Read the model definition and answer for the solid it produces. Units are mm, in the model's axes. Face numbers are marked on the shaded views. A direction names the side the tool comes from. Round coordinates to 2 decimals unless told otherwise and drop trailing zeros. Order: outer loops, then holes, each group sorted by start corner. A loop starts at its lowest first (then second) coordinate and runs counter-clockwise, first axis right, second up. Notation, with made-up numbers: (-23.75, -2.5) - (8.25, -2.5) arc R25 cw to (8.25, 16.5) - close; hole circle Ø6 at (41, 8). An arc over 180 degrees is marked (long way). Answer as a JSON object with one key per item and string values. Group by question number.
Q1. A cutting plane is placed at B-B on y = 0. Determine the outline of the cut face in (x, z).
Q2. Given pin 1 Ø3 at (x, z) = (0.5, -7) entering from -Y; pin 2 Ø1.5 at (y, z) = (-1.5, -22.5) entering from +X; pin 3 Ø1.5 at (y, z) = (1.5, -12) entering from -X, each flat-ended and moving along its own axis, determine where each tip first touches the part or whether it passes through.
Q3. A tool of negligible diameter and unlimited length cuts with its end or side. For the marked faces 1 and 2, from which of +Z, -Z, +X, -X, +Y, -Y can it reach the whole face along a straight path? Write none if from no direction.
Q4. The mould has two halves that part along Y. Classify the marked faces 3, 4 and 5: pulls with the +Y half, pulls with the -Y half, needs draft (parallel to the pull), parting line crosses it, or undercut.
Q5. Consider line 1 (Y direction, x = 0, z = -25); line 2 (Z direction, x = -0.25, y = -3); line 3 (Z direction, x = -3.5, y = 1.5). Determine where each line is inside the solid, lowest interval first.
Q6. A cutting plane is placed at D-D on z = -25. Determine the outline of the cut face in (x, y).
Q7. A cutting plane is placed at A-A on x = 0. Determine the outline of the cut face in (y, z).
Q8. A cutting plane is placed at C-C on z = -4. Determine the outline of the cut face in (x, y).
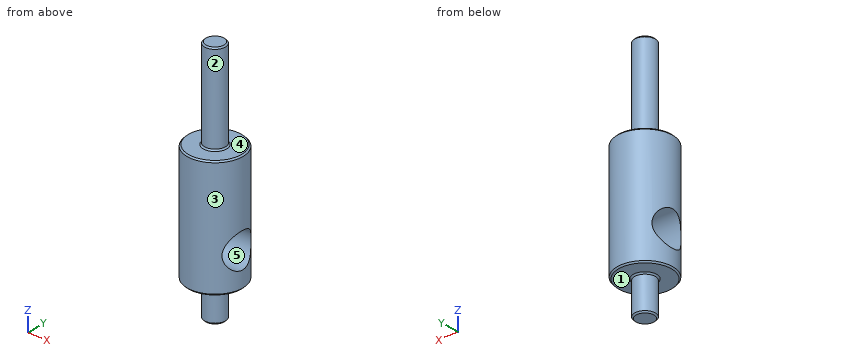
```python
from build123d import *

# Parameters (mm, degrees)
SKETCH1_R               = 1.5
BOSS_EXTRUDE1_DEPTH     = 13
SKETCH2_R               = 4
BOSS_EXTRUDE2_DEPTH     = 17
SKETCH3_R               = 1.5
BOSS_EXTRUDE3_DEPTH     = 5
CUT_EXTRUDE1_DEPTH      = 36.454195802
CUT_EXTRUDE1_DEPTH_BACK = 36.454195802
SKETCH4_R               = 2.5
CHAMFER1_SIZE           = 0.2


with BuildPart() as part:
    # Sketch1 → Boss-Extrude1 (new body)
    with BuildSketch(Plane.XY):
        Circle(SKETCH1_R)
    extrude(amount=-BOSS_EXTRUDE1_DEPTH)

    # Sketch2 → Boss-Extrude2 (add)
    with BuildSketch(Plane(origin=(0, 0, -13), x_dir=(-1, 0, 0), z_dir=(0, 0, -1))):
        Circle(SKETCH2_R)
    extrude(amount=BOSS_EXTRUDE2_DEPTH)

    # Sketch3 → Boss-Extrude3 (add)
    with BuildSketch(Plane(origin=(0, 0, -30), x_dir=(-1, 0, 0), z_dir=(0, 0, -1))):
        with Locations(Location((0, 0, 0), (0, 0, 180))):
            Circle(SKETCH3_R)
    extrude(amount=BOSS_EXTRUDE3_DEPTH)

    # Sketch4 → Cut-Extrude1 (cut, two sides: drawn at the far end of the back side and taken through both)
    with BuildSketch(Plane(origin=(0, 0, 0), x_dir=(0, 0, -1), z_dir=(1, 0, 0)).offset(-CUT_EXTRUDE1_DEPTH_BACK)):
        with Locations((25, 0)):
            Circle(SKETCH4_R)
    extrude(amount=CUT_EXTRUDE1_DEPTH + CUT_EXTRUDE1_DEPTH_BACK, mode=Mode.SUBTRACT)

    # Chamfer1
    chamfer1_edges = [part.edges().sort_by_distance(p)[0] for p in [
        (-1.5, 0, -30),
        (-1.5, 0, -35),
        (-1.5, 0, 0),
        (-1.5, 0, -13),
        (4, 0, -13),
        (4, 0, -30),
    ]]
    chamfer(chamfer1_edges, length=CHAMFER1_SIZE)


solid = part.part
```
Result set:
{
 "1": {"outline": "(-4, -29.8) - (-3.8, -30) - (-1.7, -30) - (-1.5, -30.2) - (-1.5, -34.8) - (-1.3, -35) - (1.3, -35) - (1.5, -34.8) - (1.5, -30.2) - (1.7, -30) - (3.8, -30) - (4, -29.8) - (4, -27.5) - (-4, -27.5) - close; (-4, -22.5) - (4, -22.5) - (4, -13.2) - (3.8, -13) - (1.7, -13) - (1.5, -12.8) - (1.5, -0.2) - (1.3, 0) - (-1.3, 0) - (-1.5, -0.2) - (-1.5, -12.8) - (-1.7, -13) - (-3.8, -13) - (-4, -13.2) - close"},
 "2": {"pin 1": "stops at y = -1.5", "pin 2": "stops at x = 3.93", "pin 3": "stops at x = -1.3"},
 "3": {"face 1": "-Z", "face 2": "+Z"},
 "4": {"face 3": "parting line crosses it", "face 4": "needs draft", "face 5": "undercut"},
 "5": {"line 1": "y = -4 to -2.5, 2.5 to 4", "line 2": "z = -30 to -13", "line 3": "z = -29.99 to -27, -23 to -13.01"},
 "6": {"outline": "(-3.12, -2.5) arc R4 ccw to (3.12, -2.5) - close; (-3.12, 2.5) - (3.12, 2.5) arc R4 ccw to start"},
 "7": {"outline": "(-4, -29.8) - (-3.8, -30) - (-1.7, -30) - (-1.5, -30.2) - (-1.5, -34.8) - (-1.3, -35) - (1.3, -35) - (1.5, -34.8) - (1.5, -30.2) - (1.7, -30) - (3.8, -30) - (4, -29.8) - (4, -13.2) - (3.8, -13) - (1.7, -13) - (1.5, -12.8) - (1.5, -0.2) - (1.3, 0) - (-1.3, 0) - (-1.5, -0.2) - (-1.5, -12.8) - (-1.7, -13) - (-3.8, -13) - (-4, -13.2) - close; hole circle Ø5 at (0, -25)"},
 "8": {"outline": "circle Ø3 at (0, 0)"}
}
